```python
from build123d import *

# Parameters (mm, degrees)
SKETCH1_W                = 6.8
SKETCH1_H                = 5
BOSS_EXTRUDE1_DEPTH      = 3.8
HOLE1_D                  = 1.05
HOLE1_CBORE_D            = 1.3
HOLE1_CBORE_DEPTH        = 1.2
SKETCH20_W               = 5
SKETCH20_H               = 1.3
CUT_EXTRUDE11_DEPTH      = 0.3
M1_0X0_25_TAPPED_HOLE1_D = 0.75


with BuildPart() as part:
    # Sketch1 → Boss-Extrude1 (new body)
    with BuildSketch(Plane(origin=(0, 4, 0), x_dir=(-1, 0, 0), z_dir=(0, 1, 0))):
        with Locations((-3.4, 2.5)):
            Rectangle(SKETCH1_W, SKETCH1_H)
    extrude(amount=-BOSS_EXTRUDE1_DEPTH)

    # Hole1 (through all)
    with Locations(Plane(origin=(0, 0, 0), x_dir=(-1, 0, 0), z_dir=(0, 0, -1))):
        with Locations((-5.7, 1.7), (-0.7, 1.7)):
            CounterBoreHole(HOLE1_D / 2, HOLE1_CBORE_D / 2, HOLE1_CBORE_DEPTH)

    # Sketch20 → Cut-Extrude11 (cut)
    with BuildSketch(Plane(origin=(6.8, 0, 0), x_dir=(0, 0, -1), z_dir=(1, 0, 0))):
        with Locations((-2.5, 3.35)):
            Rectangle(SKETCH20_W, SKETCH20_H)
    extrude(amount=-CUT_EXTRUDE11_DEPTH, mode=Mode.SUBTRACT)

    # M1.0x0.25 Tapped Hole1 (through all)
    with Locations(Plane(origin=(0, 0, 0), x_dir=(-1, 0, 0), z_dir=(0, 0, -1))):
        with Locations((-3.2, 1.7)):
            Hole(M1_0X0_25_TAPPED_HOLE1_D / 2)


solid = part.part
```
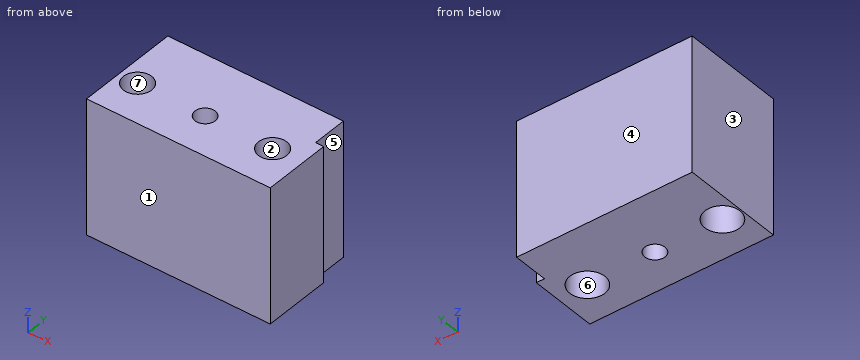
Verification items for the finished model (mm, model axes). Face numbers are marked on the shaded views. A direction names the side the tool comes from. Coordinates: 2 decimals unless noted, no trailing zeros. Loops run counter-clockwise (first coordinate to the right, second up) from the corner with the lowest first, then second, coordinate; pieces in that order, holes last. Notation, with made-up numbers: (8, 59) -> (44, 59) arc R21 ccw to (44, 89) -> close; hole circle Ø9 at (18.5, 88.25). An arc over 180 degrees is marked (long way). Answer in a Markdown table with one row per item. Add a question column.
1. Depth check by flat-ended pin: P1, Ø0.8, axis at x = 5.7, y = 1.7, coming from the +Z side; P2, Ø1, axis at y = 3.5, z = 4, coming from the +X side; P3, Ø1.2, axis at x = 0.7, y = 1.7, coming from the -Z side. Enter the tip coordinate at first touch or a pass-through.
2. Material ranges on probe 1 along Y at (x, z) = (5.7, 3.95) (3 decimals); probe 2 along Y at (x, z) = (5.7, 0.5); probe 3 along X at (y, z) = (3.2, 0.65), recorded low to high. Write a range as [from, to].
3. Access from +Z, -Z, +X, -X, +Y, -Y to the whole of each face (thin tool, end or side, straight path). Record for the marked faces 5, 6 and 7.
4. Draft check along Y on the marked faces 1, 2, 3 and 4. Enter one of: +Y half, -Y half, draft (parallel to the pull), parting line (faces both ways), or undercut.
5. Section check A-A, the plane y = 1.7. Enter the section's corners in (x, z) (3 decimals), then the cut area to 4 significant figures.
6. Section check C-C, the plane z = 4.15. Enter the section's corners in (x, y) (3 decimals), then the cut area to 3 significant figures.
7. Section check B-B, the plane x = 5.7. Enter the section's corners in (y, z) (3 decimals).
8. Section check D-D, the plane x = 3.2. Enter the section's corners in (y, z) (3 decimals).
Derived:
| question | item | result |
|---|---|---|
| 1 | P1 | passes through |
| 1 | P2 | stops at x = 6.5 |
| 1 | P3 | stops at z = 1.2 |
| 2 | probe 1 | y = [0.2, 1.175], [2.225, 4] |
| 2 | probe 2 | y = [0.2, 1.05], [2.35, 4] |
| 2 | probe 3 | x = [0, 6.5] |
| 3 | face 5 | +Z, -Z, +X, +Y |
| 3 | face 6 | -Z |
| 3 | face 7 | +Z, -Z |
| 4 | face 1 | -Y half |
| 4 | face 2 | undercut |
| 4 | face 3 | draft |
| 4 | face 4 | +Y half |
| 5 | outline | (0, 0) -> (0.05, 0) -> (0.05, 1.2) -> (0.175, 1.2) -> (0.175, 5) -> (0, 5) -> close; (1.225, 1.2) -> (1.35, 1.2) -> (1.35, 0) -> (2.825, 0) -> (2.825, 5) -> (1.225, 5) -> close; (3.575, 0) -> (5.05, 0) -> (5.05, 1.2) -> (5.175, 1.2) -> (5.175, 5) -> (3.575, 5) -> close; (6.225, 1.2) -> (6.35, 1.2) -> (6.35, 0) -> (6.8, 0) -> (6.8, 5) -> (6.225, 5) -> close |
| 5 | area | 19.15 mm² |
| 6 | outline | (0, 0.2) -> (6.8, 0.2) -> (6.8, 2.7) -> (6.5, 2.7) -> (6.5, 4) -> (0, 4) -> close; hole circle Ø1.05 at (0.7, 1.7); hole circle Ø0.75 at (3.2, 1.7); hole circle Ø1.05 at (5.7, 1.7) |
| 6 | area | 23.3 mm² |
| 7 | outline | (0.2, 0) -> (1.05, 0) -> (1.05, 1.2) -> (1.175, 1.2) -> (1.175, 5) -> (0.2, 5) -> close; (2.225, 1.2) -> (2.35, 1.2) -> (2.35, 0) -> (4, 0) -> (4, 5) -> (2.225, 5) -> close |
| 8 | outline | (0.2, 0) -> (1.325, 0) -> (1.325, 5) -> (0.2, 5) -> close; (2.075, 0) -> (4, 0) -> (4, 5) -> (2.075, 5) -> close |
